Input: part model. Units: mm. Frame: model coordinates. A direction names the side the tool comes from. Coordinates: 2 decimals unless noted, no trailing zeros. Order: outer loops, then holes, each group sorted by start corner. A loop starts at its lowest first (then second) coordinate and runs counter-clockwise, first axis right, second up. Notation, with made-up numbers: M 20.5,1 L 78.5,1 A29 ccw 78.5,35 Z; hole C 79.25,78.5 d2. An arc over 180 degrees is marked long. Answer in a Markdown table with one row per item.
Autodesk Inventor part; units mm, degrees
ref_plane "YZ Plane" through (0, 0, 0) normal (1, 0, 0) x (0, 1, 0)
ref_plane "XZ Plane" through (0, 0, 0) normal (0, 1, 0) x (-1, 0, 0)
ref_plane "XY Plane" through (0, 0, 0) normal (0, 0, 1) x (1, 0, 0)
sketch "Эскиз1" plane through (0, 0, 0) normal (0, 1, 0) x (-1, 0, 0)
  circle A0 centre (0, 0) radius 1.35
  line L0 (0.5, -3.5) -> (-48.5, -3.5)
  arc A1 (-51.5, -0.5) -> (-48.5, -3.5) centre (-48.5, -0.5) ccw
  line L1 (-51.5, -0.5) -> (-51.5, 33.5)
  arc A2 (-48.5, 36.5) -> (-51.5, 33.5) centre (-48.5, 33.5) ccw
  line L2 (-48.5, 36.5) -> (0.5, 36.5)
  arc A3 (3.5, 33.5) -> (0.5, 36.5) centre (0.5, 33.5) ccw
  line L3 (3.5, 33.5) -> (3.5, -0.5)
  arc A4 (0.5, -3.5) -> (3.5, -0.5) centre (0.5, -0.5) ccw
  circle A5 centre (-48, 33) radius 1.35
  circle A6 centre (0, 33) radius 1.35
  circle A7 centre (-48, 0) radius 1.35
  circle A8 centre (0, 0) radius 1.35
  line L4 (-48.5, -3.8) -> (0.5, -3.8)
  arc A9 (0.5, -3.8) -> (3.8, -0.5) centre (0.5, -0.5) ccw
  line L5 (3.8, -0.5) -> (3.8, 33.5)
  arc A10 (3.8, 33.5) -> (0.5, 36.8) centre (0.5, 33.5) ccw
  line L6 (0.5, 36.8) -> (-48.5, 36.8)
  arc A11 (-48.5, 36.8) -> (-51.8, 33.5) centre (-48.5, 33.5) ccw
  line L7 (-51.8, 33.5) -> (-51.8, -0.5)
  arc A12 (-51.8, -0.5) -> (-48.5, -3.8) centre (-48.5, -0.5) ccw
  circle A13 centre (0, 0) radius 3.5
  line L8 (1.6675, -3.0773) -> (12.7, 2.901)
  line L9 (10.5, 14.101) -> (6, 14.101)
  line L10 (6, 14.101) -> (6, 5.101)
  line L11 (6, 5.101) -> (10.5, 5.101)
  line L12 (10.5, 5.101) -> (10.5, 14.101)
  line L13 (5.8, 4.901) -> (5.8, 14.301)
  line L14 (5.8, 14.301) -> (10.7, 14.301)
  line L15 (10.7, 14.301) -> (10.7, 4.901)
  line L16 (10.7, 4.901) -> (5.8, 4.901)
  line L17 (3.8, 2.901) -> (3.8, 16.301)
  line L18 (3.8, 16.301) -> (12.7, 16.301)
  line L19 (12.7, 16.301) -> (12.7, 2.901)
  line L20 (12.7, 2.901) -> (3.8, 2.901)
  line L21 (-3.1671, 1.4898) -> (3.8, 16.301)
  line L22 (19.4615, 18.801) -> (-3.6385, 18.801)
  dimension "d0" = 2.7
  dimension "d1" = 0.3
  dimension "d2" = 7
  dimension "d3" = 4.5
  dimension "d4" = 9
  dimension "d5" = 0.2
  dimension "d6" = 2
  dimension "d7" = 2.5
extrude "Выдавливание1" add sketch "Эскиз1" against normal blind 2 contours A13 | L8 A13 L3 A4 | A4 L3 L21 L5 A9 L8 | L21 L3 A13 | A9 L5 L20 L8 | L20 L5 L18 L19
chamfer "Фаска1" distance 1 angle 45 1 edges at (1.35, -2, 0)
fillet "Сопряжение1" radius 1.5 3 edges at (-12.7, -1, 2.901) (-3.8, -1, 16.301) (-12.7, -1, 16.301)
sketch "Эскиз2" plane through (0, 0, 0) normal (0, 1, 0) x (1, 0, 0)
  line L0 (-0.5, 3.5) -> (48.5, 3.5)
  arc A0 (51.5, 0.5) -> (48.5, 3.5) centre (48.5, 0.5) ccw
  line L1 (51.5, 0.5) -> (51.5, -33.5)
  arc A1 (48.5, -36.5) -> (51.5, -33.5) centre (48.5, -33.5) ccw
  line L2 (48.5, -36.5) -> (-0.5, -36.5)
  arc A2 (-3.5, -33.5) -> (-0.5, -36.5) centre (-0.5, -33.5) ccw
  line L3 (-3.5, -33.5) -> (-3.5, 0.5)
  arc A3 (-0.5, 3.5) -> (-3.5, 0.5) centre (-0.5, 0.5) ccw
  circle A4 centre (48, -33) radius 1.35
  circle A5 centre (0, -33) radius 1.35
  circle A6 centre (48, 0) radius 1.35
  circle A7 centre (0, 0) radius 1.35
  line L4 (48.5, 4) -> (-0.5, 4)
  arc A8 (-0.5, 4) -> (-4, 0.5) centre (-0.5, 0.5) ccw
  line L5 (-4, 0.5) -> (-4, -33.5)
  arc A9 (-4, -33.5) -> (-0.5, -37) centre (-0.5, -33.5) ccw
  line L6 (-0.5, -37) -> (48.5, -37)
  arc A10 (48.5, -37) -> (52, -33.5) centre (48.5, -33.5) ccw
  line L7 (52, -33.5) -> (52, 0.5)
  arc A11 (52, 0.5) -> (48.5, 4) centre (48.5, 0.5) ccw
  arc A12 (-12.7, -14.801) -> (-11.2, -16.301) centre (-11.2, -14.801) ccw
  line L8 (-11.2, -16.301) -> (-4.7521, -16.301)
  arc A13 (-4.7521, -16.301) -> (-3.3947, -15.4395) centre (-4.7521, -14.801) ccw
  line L9 (-3.3947, -15.4395) -> (3.1671, -1.4898)
  arc A14 (3.1671, -1.4898) -> (-1.6675, 3.0773) centre (0, 0) ccw
  line L10 (-1.6675, 3.0773) -> (-11.9146, -2.4754)
  arc A15 (-11.9146, -2.4754) -> (-12.7, -3.7943) centre (-11.2, -3.7943) ccw
  line L11 (-12.7, -3.7943) -> (-12.7, -14.801)
  circle A16 centre (0, 0) radius 1.35
  line L12 (-5.8, -4.901) -> (-5.8, -14.301)
  line L13 (-5.8, -14.301) -> (-10.7, -14.301)
  line L14 (-10.7, -14.301) -> (-10.7, -4.901)
  line L15 (-10.7, -4.901) -> (-5.8, -4.901)
  point P0 (-4, -16.0988)
  point P1 (-3.6646, 1.9951)
  dimension "d6" = 2
  dimension "d14" = 0.5
extrude "Выдавливание2" add sketch "Эскиз2" along normal blind 1 contours A8 L5 A13 L8 A12 L11 A15 L10 | L12 L13 L14 L15
properties part number "bonnet_fixator"
1) Cut plane A-A, the plane y = -0.35. Output: boundary loops of the cut face in (x, z), and give its area (3 significant figures).
Resolved:
| item | result |
|---|---|
| outline | M -12.7,3.79 A1.5 ccw -11.91,2.48 L -1.67,-3.08 A3.5 ccw 3.17,1.49 L -3.39,15.44 A1.5 ccw -4.75,16.3 L -11.2,16.3 A1.5 ccw -12.7,14.8 Z; hole M -10.7,4.9 L -5.8,4.9 L -5.8,14.3 L -10.7,14.3 Z; hole C 0,0 d2.7 |
| area | 171 mm2 |
2) Cut plane D-D, the plane x = -6.75. Output: boundary loops of the cut face in (y, z), and give its area (3 significant figures).
Resolved:
| item | result |
|---|---|
| outline | M -2,-0.32 L 1,-0.32 L 1,16.3 L -2,16.3 L -2,14.3 L 0,14.3 L 0,4.9 L -2,4.9 Z |
| area | 31.1 mm2 |
3) Reachability of faces 1 (the face through (-3.917, 0.493, -1.256)), 2 (the face through (-8, 0, 16.301)), 3 (the face through (-8, -1, 4.901)) from +Z, -Z, +X, -X, +Y, -Y: full face, straight path, thin tool, end or side. Return the list, or none.
Resolved:
| item | result |
|---|---|
| face 1 | +Z, +X, +Y |
| face 2 | +Z, +X, -X, +Y, -Y |
| face 3 | -Y |
4) Mould query, pull axis X, two halves, no side actions, for faces 4 (the face through (-4, 0.5, 7.7)), 5 (the face through (-5.8, -1, 10)), 6 (the face through (2.45, -0.99, -2.5)), 7 (the face through (-8, -1, 14.301)). Classes: +X half, -X half, draft (parallel to the pull), parting line (faces both ways), or undercut.
Resolved:
| item | result |
|---|---|
| face 4 | +X half |
| face 5 | undercut |
| face 6 | parting line |
| face 7 | undercut |
5) Cut plane B-B, the plane z = 0. Output: boundary loops of the cut face in (x, y), and give its area (3 significant figures).
Resolved:
| item | result |
|---|---|
| outline | M -7.35,-2 L -2.35,-2 L -1.35,-1 L -1.35,0 L -4,0 L -4,1 L -7.35,1 Z; M 1.35,-1 L 2.35,-2 L 3.5,-2 L 3.5,0 L 1.35,0 Z |
| area | 18.6 mm2 |
6) Material intervals for probe 1 along Y at (x, z) = (-2.5, 6.75); probe 2 along Z at (x, y) = (0, -0.6); probe 3 along X at (y, z) = (-0.7, 1), sorted ascending.
Resolved:
| item | result |
|---|---|
| probe 1 | y = -2 to 0 |
| probe 2 | z = -3.5 to -1.35, 1.35 to 8.22 |
| probe 3 | x = -9.19 to -0.91, 0.91 to 3.35 |
7) Cut plane C-C, the plane y = -1.5. Output: boundary loops of the cut face in (x, z).
Resolved:
| item | result |
|---|---|
| outline | M -12.7,3.79 A1.5 ccw -11.91,2.48 L -1.67,-3.08 A3.5 ccw 3.17,1.49 L -3.39,15.44 A1.5 ccw -4.75,16.3 L -11.2,16.3 A1.5 ccw -12.7,14.8 Z; hole M -10.7,4.9 L -5.8,4.9 L -5.8,14.3 L -10.7,14.3 Z; hole C 0,0 d3.7 |
8) Contact query for flat-ended pins moving along their axis: pin 1 (1.6 mm diameter, centred on y = -1, z = 8, fed in from +X); pin 2 (4 mm diameter, centred on x = -1, z = -1.5, fed in from +Y). Output: stop coordinate, or through.
Resolved:
| item | result |
|---|---|
| pin 1 | stops at x = 0.48 |
| pin 2 | stops at y = 0 |
